Check sheet for the modelled part. Datum: model origin and axes. Units: mm. Face numbers are marked on the shaded views. A direction names the side the tool comes from. Give positions to 0.01 mm unless a question says otherwise; leave off trailing zeros. Write each loop counter-clockwise with the first axis right and the second up, starting at its lowest first coordinate (ties: lowest second). Pieces come first, ordered by that corner, then holes. Notation, with made-up numbers: M 49,-40 L 55,-40 A4 ccw 55,-36 Z; hole C 55,-11 d11. An arc over 180 degrees is marked long. Write item = value, one per line. Start each with the question number.
1) Scan lines: L1, parallel to Z at x = 38, y = 3.85; L2, parallel to X at y = 3.6, z = 105; L3, parallel to Z at x = 3.85, y = 44. Record each from-to range of solid material in increasing order.
2) Sectioned sample at C-C, the plane y = 44. Record the cut outline in (x, z).
3) Sectioned sample at B-B, the plane z = 0. Record the cut outline in (x, y), then the cut area to 3 significant figures.
4) Gauge pin test, flat ends, axial feed: pin 1 (21 mm diameter, centred on x = 38, z = -60, fed in from -Y); pin 2 (8 mm diameter, centred on x = 38, z = 60, fed in from +Y); pin 3 (2 mm diameter, centred on x = 21.5, z = 95.5, fed in from +Y); pin 4 (8 mm diameter, centred on y = 70.5, z = 92.5, fed in from +X). Record the tip position at first contact, or that the pin passes through.
5) Sectioned sample at A-A, the plane x = 38. Record the cut outline in (y, z), then the cut area to 3 significant figures.
6) Set-up check for the marked faces 1 and 2: record each of +Z, -Z, +X, -X, +Y, -Y from which the full face is reachable in a straight line by a thin tool's end or side.
7) Sectioned sample at D-D, the plane z = 48.5. Record the cut outline in (x, y).
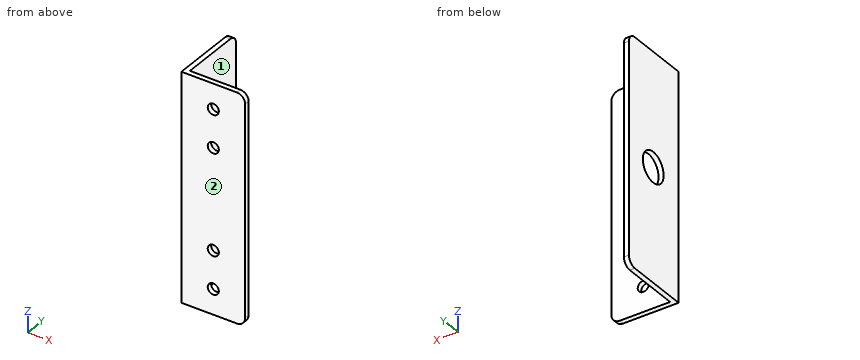
from build123d import *

# Parameters (mm, degrees)
EXTRUDE_1_DEPTH     = 135
SKETCH_3_R          = 18
CUT_EXTRUDE_2_DEPTH = 175.702604445
SKETCH_4_R          = 6.6
CUT_EXTRUDE_3_DEPTH = 175.358825415
FILLET_1_R          = 10


with BuildPart() as part:
    # Эскиз1 → Бобышка-Вытянуть1 (new, symmetric)
    with BuildSketch(Plane.XY):
        Polygon((0, 0), (76, 0), (76, 6), (6, 6), (6, 86), (0, 86), align=None)
    extrude(amount=EXTRUDE_1_DEPTH, both=True)

    # Эскиз3 → Вырез-Вытянуть2 (cut, through all)
    with BuildSketch(Plane(origin=(6, 0, 0), x_dir=(0, 0, -1), z_dir=(1, 0, 0))):
        with Locations(Location((0, 44, 0), (0, 0, 90))):
            Circle(SKETCH_3_R)
    extrude(amount=-CUT_EXTRUDE_2_DEPTH, mode=Mode.SUBTRACT)

    # Эскиз4 → Вырез-Вытянуть3 (cut, through all)
    with BuildSketch(Plane(origin=(0, 6, 0), x_dir=(1, 0, 0), z_dir=(0, 1, 0))):
        with Locations(Location((38, 105, 0), (0, 0, 180))):
            Circle(SKETCH_4_R)
        with Locations((38, 60)):
            Circle(SKETCH_4_R)
        with Locations(Location((38, -60, 0), (0, 0, 180))):
            Circle(SKETCH_4_R)
        with Locations((38, -105)):
            Circle(SKETCH_4_R)
    extrude(amount=-CUT_EXTRUDE_3_DEPTH, mode=Mode.SUBTRACT)

    # Скругление1
    fillet_1_edges = [part.edges().sort_by_distance(p)[0] for p in [
        (76, 3, 135),
        (3, 86, 135),
        (3, 86, -135),
        (76, 3, -135),
    ]]
    fillet(fillet_1_edges, radius=FILLET_1_R)


solid = part.part
Data:
q1.L1 = -135 to -111.6, -98.4 to -66.6, -53.4 to 53.4, 66.6 to 98.4, 111.6 to 135
q1.L2 = 0 to 31.4, 44.6 to 76
q1.L3 = -135 to -18, 18 to 135
q2.outline = M 0,-135 L 6,-135 L 6,-18 L 0,-18 Z; M 0,18 L 6,18 L 6,135 L 0,135 Z
q3.outline = M 0,0 L 76,0 L 76,6 L 6,6 L 6,26 L 0,26 Z; M 0,62 L 6,62 L 6,86 L 0,86 Z
q3.area = 720 mm2
q4.pin_1 = 0
q4.pin_2 = through
q4.pin_3 = 6
q4.pin_4 = 6
q5.outline = M 0,-135 L 6,-135 L 6,-111.6 L 0,-111.6 Z; M 0,-98.4 L 6,-98.4 L 6,-66.6 L 0,-66.6 Z; M 0,-53.4 L 6,-53.4 L 6,53.4 L 0,53.4 Z; M 0,66.6 L 6,66.6 L 6,98.4 L 0,98.4 Z; M 0,111.6 L 6,111.6 L 6,135 L 0,135 Z
q5.area = 1,300 mm2
q6.face_1 = +Z, -Z, +X, +Y
q6.face_2 = +Z, -Z, +X, -X, -Y
q7.outline = M 0,0 L 76,0 L 76,6 L 6,6 L 6,86 L 0,86 Z
